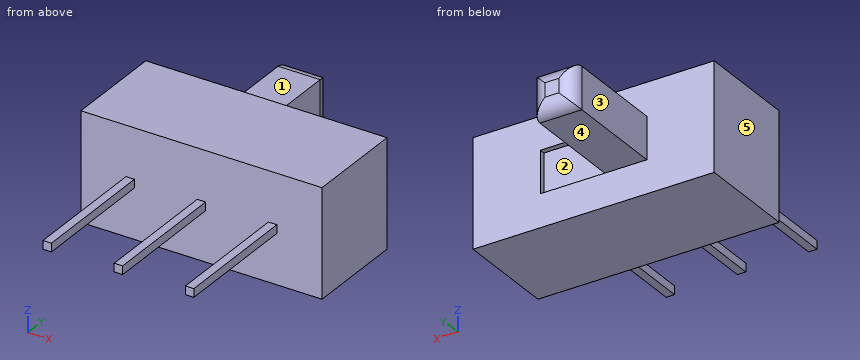
```python
from build123d import *

# Parameters (mm, degrees)
SKETCH2_W           = 8.6
SKETCH2_H           = 3.85
BOSS_EXTRUDE1_DEPTH = 3.6
SKETCH3_W           = 1.5
SKETCH3_H           = 1.5
BOSS_EXTRUDE2_DEPTH = 4.1
SKETCH4_W           = 2.3
SKETCH4_H           = 1.5
CUT_EXTRUDE1_DEPTH  = 0.2
FILLET1_R           = 0.5
SKETCH5_W           = 0.3
SKETCH5_H           = 0.3
BOSS_EXTRUDE3_DEPTH = 4.6


with BuildPart() as part:
    # Sketch2 → Boss-Extrude1 (new body)
    with BuildSketch(Plane(origin=(0, 0, 0), x_dir=(1, 0, 0), z_dir=(0, 1, 0))):
        Rectangle(SKETCH2_W, SKETCH2_H)
    extrude(amount=BOSS_EXTRUDE1_DEPTH)

    # Sketch3 → Boss-Extrude2 (add)
    with BuildSketch(Plane(origin=(0, 3.6, 0), x_dir=(1, 0, 0), z_dir=(0, 1, 0))):
        with Locations((-1.15, 0)):
            Rectangle(SKETCH3_W, SKETCH3_H)
    extrude(amount=BOSS_EXTRUDE2_DEPTH)

    # Sketch4 → Cut-Extrude1 (cut)
    with BuildSketch(Plane(origin=(0, 3.6, 0), x_dir=(1, 0, 0), z_dir=(0, 1, 0))):
        with Locations((0.75, 0)):
            Rectangle(SKETCH4_W, SKETCH4_H)
    extrude(amount=-CUT_EXTRUDE1_DEPTH, mode=Mode.SUBTRACT)

    # Fillet1
    fillet1_edges = [part.edges().sort_by_distance(p)[0] for p in [
        (-0.4, 7.7, 0),
        (-1.15, 7.7, -0.75),
        (-1.9, 7.7, 0),
        (-1.15, 7.7, 0.75),
    ]]
    fillet(fillet1_edges, radius=FILLET1_R)

    # Sketch5 → Boss-Extrude3 (add)
    with BuildSketch(Plane.XZ):
        Rectangle(SKETCH5_W, SKETCH5_H)
        with Locations((-2.54, 0)):
            Rectangle(SKETCH5_W, SKETCH5_H)
        with Locations((2.54, 0)):
            Rectangle(SKETCH5_W, SKETCH5_H)
    extrude(amount=BOSS_EXTRUDE3_DEPTH)


solid = part.part
```
Geometry check sheet. Reference: the model listing, model coordinates, mm. Face numbers are marked on the shaded views. A direction names the side the tool comes from. Coordinates: 2 decimals unless noted, no trailing zeros. Order: outer loops, then holes, each group sorted by start corner. A loop starts at its lowest first (then second) coordinate and runs counter-clockwise, first axis right, second up.
Item 1: Depth check by flat-ended pin: pin 1 (1.6 mm diameter, centred on x = -1, y = 5, fed in from -Z); pin 2 (0.8 mm diameter, centred on y = 5.5, z = 0, fed in from +X); pin 3 (1.6 mm diameter, centred on y = 5, z = -0.5, fed in from -X). Enter the tip coordinate at first touch or a pass-through.
Item 2: Tool access check on the marked faces 1, 2, 3, 4 and 5. Record the directions out of +Z, -Z, +X, -X, +Y, -Y that give a thin tool (end or side, any length) a straight path to the whole face; none if there is none.
Item 3: Scan lines: line 1 along Z through (x, y) = (1, 3.5) (3 decimals); line 2 along Y through (x, z) = (-2.5, -0.5); line 3 along X through (y, z) = (6.5, 0.6). Record each from-to range of solid material in increasing order.
Item 4: Section check B-B (x = -1.25). Enter the section's corners in (y, z) (3 decimals).
Item 5: Section check D-D (x = 0). Enter the section's corners in (y, z) (3 decimals), plus the area to 3 significant figures.
Item 6: Section check A-A (y = -3.25). Enter the section's corners in (x, z).
Item 7: Section check C-C (z = -0.55). Enter the section's corners in (x, y), plus the area to 3 significant figures.
Check sheet entries:
1. pin 1: stops at z = -0.75
1. pin 2: stops at x = -0.4
1. pin 3: stops at x = -1.9
2. face 1: +Z, +X, -X, +Y
2. face 2: +Y
2. face 3: +Z, -Z, -X, +Y
2. face 4: -Z, +X, -X, +Y
2. face 5: +Z, -Z, -X, +Y, -Y
3. line 1: z = -1.925 to -0.75, 0.75 to 1.925
3. line 2: y = 0 to 3.6
3. line 3: x = -1.9 to -0.4
4. outline: (0, -1.925) - (3.6, -1.925) - (3.6, -0.75) - (7.2, -0.75) arc R0.5 ccw to (7.7, -0.25) - (7.7, 0.25) arc R0.5 ccw to (7.2, 0.75) - (3.6, 0.75) - (3.6, 1.925) - (0, 1.925) - close
5. outline: (-4.6, -0.15) - (0, -0.15) - (0, -1.925) - (3.6, -1.925) - (3.6, -0.75) - (3.4, -0.75) - (3.4, 0.75) - (3.6, 0.75) - (3.6, 1.925) - (0, 1.925) - (0, 0.15) - (-4.6, 0.15) - close
5. area: 14.9 mm2
6. outline: (-2.69, -0.15) - (-2.39, -0.15) - (-2.39, 0.15) - (-2.69, 0.15) - close; (-0.15, -0.15) - (0.15, -0.15) - (0.15, 0.15) - (-0.15, 0.15) - close; (2.39, -0.15) - (2.69, -0.15) - (2.69, 0.15) - (2.39, 0.15) - close
7. outline: (-4.3, 0) - (4.3, 0) - (4.3, 3.6) - (1.9, 3.6) - (1.9, 3.4) - (-0.4, 3.4) - (-0.4, 7.2) arc R0.5 ccw to (-0.6, 7.6) - (-1.7, 7.6) arc R0.5 ccw to (-1.9, 7.2) - (-1.9, 3.6) - (-4.3, 3.6) - close
7. area: 36.5 mm2
